Check sheet for the modelled part. Datum: model origin and axes. Units: mm. Face numbers are marked on the shaded views. A direction names the side the tool comes from. Round coordinates to 2 decimals unless told otherwise and drop trailing zeros. Loops run counter-clockwise (first coordinate to the right, second up) from the corner with the lowest first, then second, coordinate; pieces in that order, holes last. Notation, with made-up numbers: (83.25, 32.25) -> (136.25, 32.25) arc R6 ccw to (136.25, 37.25) -> close; hole circle Ø2 at (-5.75, 65.5). An arc over 180 degrees is marked (long way). Use one line per item in the form item = value. Start each with the question number.
(1) Material ranges on probe 1 along Z at (x, y) = (20, -8); probe 2 along Z at (x, y) = (39.5, -37); probe 3 along Y at (x, z) = (27.5, 34), recorded low to high. Write a range as [from, to].
(2) Sectioned sample at D-D (x = 4). Record the cut outline in (y, z), and give its area (3 significant figures).
(3) Sectioned sample at B-B (z = 24.5). Record the cut outline in (x, y).
(4) Sectioned sample at C-C (x = 13.5). Record the cut outline in (y, z).
(5) Go/stop test with flat-tipped pins: pin 1 (8 mm diameter, centred on x = 42.5, y = -11, fed in from +Z); pin 2 (1.5 mm diameter, centred on y = -13, z = 15, fed in from +X); pin 3 (24 mm diameter, centred on x = 35.5, z = 24, fed in from -Y); pin 4 (12 mm diameter, centred on y = -28.5, z = 31.5, fed in from +X). Record where each tip stops, or that it passes through.
(6) Set-up check for the marked faces 1, 2 and 3: record each of +Z, -Z, +X, -X, +Y, -Y from which the full face is reachable in a straight line by a thin tool's end or side.
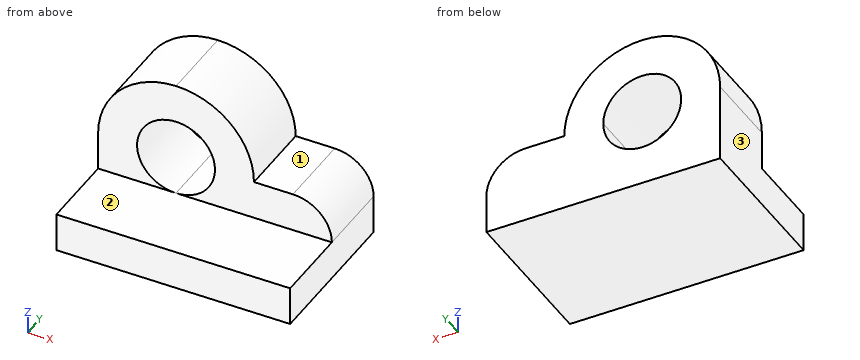
from build123d import *

# Parameters (mm, degrees)
F0_W     = 60
F0_H     = 10
F1_DEPTH = 40
F2_W     = 20
F2_H     = 20
F3_DEPTH = 10
F4_W     = 40
F4_H     = 20
F5_DEPTH = 30
F6_R     = 10
F7_R     = 19.99999
F9_DEPTH = 25


# Not quite as in the source:
# - a fillet or chamfer is up to 0.001 mm smaller than in the source, because OpenCascade refuses the exact size


with BuildPart() as f1:
    # F0 (on Front) → F1 (new body)
    with BuildSketch(Plane.XZ):
        with Locations((30, 5)):
            Rectangle(F0_W, F0_H)
    extrude(amount=F1_DEPTH)

    # F2 (on face) → F3 (join)
    with BuildSketch(Plane.XY.offset(10)):
        with Locations((50, -10)):
            Rectangle(F2_W, F2_H)
    extrude(amount=F3_DEPTH)

    # F4 (on face) → F5 (join)
    with BuildSketch(Plane.XY.offset(10)):
        with Locations((20, -10)):
            Rectangle(F4_W, F4_H)
    extrude(amount=F5_DEPTH)

    # F6
    f6_edges = [f1.edges().sort_by_distance(p)[0] for p in [
        (60, -10, 20),
    ]]
    fillet(f6_edges, radius=F6_R)

    # F7 (radius 20 in the source; OpenCascade refuses exactly that, so slightly less here)
    f7_edges = [f1.edges().sort_by_distance(p)[0] for p in [
        (40, -10, 40),
        (0, -10, 40),
    ]]
    fillet(f7_edges, radius=F7_R)

    # F8 (on face) → F9 (cut)
    with BuildSketch(Plane.XZ.offset(20)):
        with BuildLine():
            ThreePointArc((20, 10), (27.0710678119, 12.9289321881), (30, 20))
            ThreePointArc((30, 20), (12.9289321881, 27.0710678119), (20, 10))
        make_face()
    extrude(amount=-F9_DEPTH, mode=Mode.SUBTRACT)


solid = f1.part
Checks:
q1.probe_1 = [0, 10], [30, 40]
q1.probe_2 = [0, 10]
q1.probe_3 = [-20, 0]
q2.outline = (-40, 0) -> (0, 0) -> (0, 32) -> (-20, 32) -> (-20, 10) -> (-40, 10) -> close
q2.area = 840 mm2
q3.outline = (0.51, -20) -> (11.07, -20) -> (11.07, 0) -> (0.51, 0) -> close; (28.93, -20) -> (39.49, -20) -> (39.49, 0) -> (28.93, 0) -> close
q4.outline = (-40, 0) -> (0, 0) -> (0, 12.4) -> (-20, 12.4) -> (-20, 10) -> (-40, 10) -> close; (-20, 27.6) -> (0, 27.6) -> (0, 38.91) -> (-20, 38.91) -> close
q5.pin_1 = 27.6
q5.pin_2 = 59.05
q5.pin_3 = -20
q5.pin_4 = through
q6.face_1 = +Z, +X, +Y, -Y
q6.face_2 = +Z, +X, -X, -Y
q6.face_3 = +Z, -Z, -X, +Y, -Y
